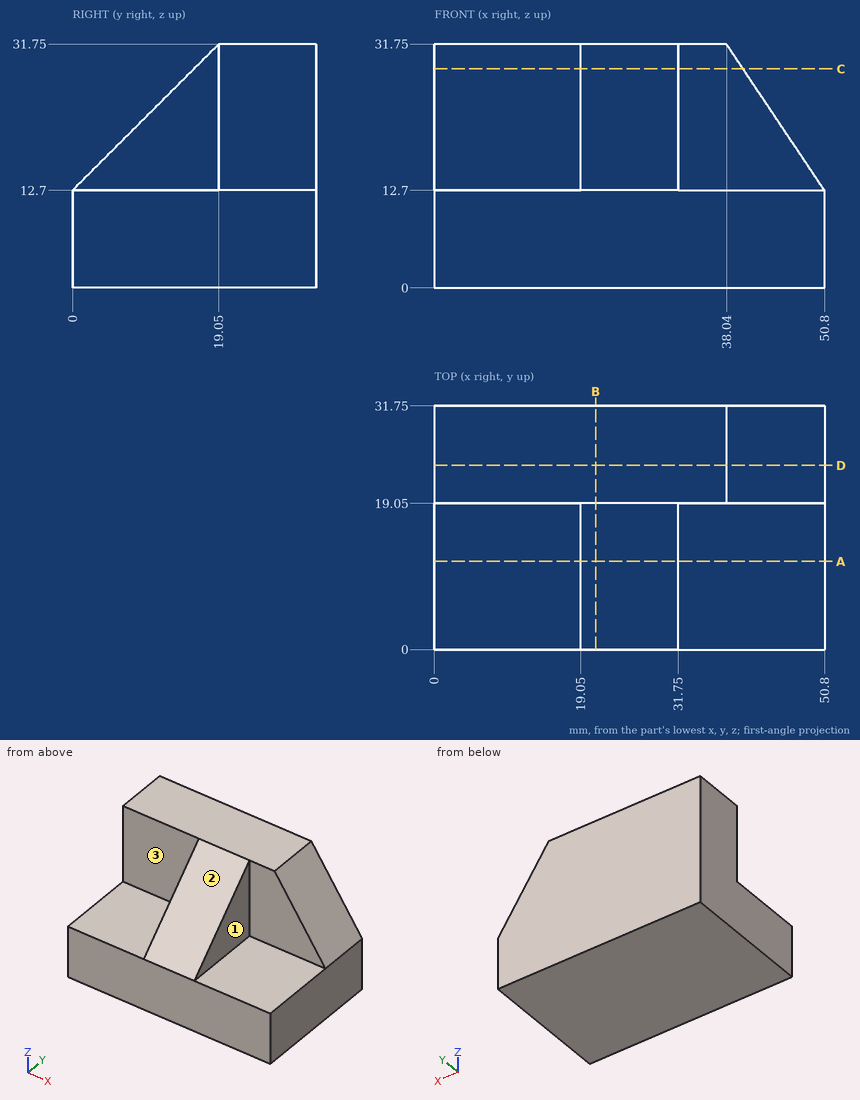
Job drawing, mm, ordinate dimensions from the low corner. One solid piece. A direction names the side the tool comes from. Coordinates: 2 decimals unless noted, no trailing zeros. Write each loop counter-clockwise with the first axis right and the second up, starting at its lowest first coordinate (ties: lowest second). Pieces come first, ordered by that corner, then holes.
Item 1: Pin check, flat tips, straight feed: pin 1 (3 mm diameter, centred on x = 5.5, y = 7, fed in from +Z); pin 2 (9.5 mm diameter, centred on x = 40, z = 20, fed in from -Y); pin 3 (1.5 mm diameter, centred on y = 6.5, z = 13.5, fed in from +X). Stop position of each tip, or through.
Item 2: Which spindle directions (+Z, -Z, +X, -X, +Y, -Y) get a long thin tool onto all of the face, cutting with end or side? Do the marked faces 1, 2 and 3. Say none if no direction does.
Item 3: Slice it at A-A (y = 11.5). Write the cut outline in (x, z), and give its area (3 significant figures).
Item 4: Probe line 1 (Z direction, x = 37.5, y = 8); line 2 (X direction, y = 3.5, z = 15). List the from-to ranges inside material, lowest first.
Item 5: Slice it at C-C (z = 28.5). Write the cut outline in (x, y).
Item 6: Slice it at B-B (x = 21). Write the cut outline in (y, z), and give its area (3 significant figures).
Item 7: Slice it at D-D (y = 24). Write the cut outline in (x, z).
Results found:
1. pin 1: stops at z = 12.7
1. pin 2: stops at y = 19.05
1. pin 3: stops at x = 31.75
2. face 1: +Z, +X, -Y
2. face 2: +Z, +X, -X, -Y
2. face 3: +Z, -X, -Y
3. outline: (0, 0) - (50.8, 0) - (50.8, 12.7) - (31.75, 12.7) - (31.75, 24.2) - (19.05, 24.2) - (19.05, 12.7) - (0, 12.7) - close
3. area: 791 mm2
4. line 1: z = 0 to 12.7
4. line 2: x = 19.05 to 31.75
5. outline: (0, 19.05) - (19.05, 19.05) - (19.05, 15.8) - (31.75, 15.8) - (31.75, 19.05) - (40.22, 19.05) - (40.22, 31.75) - (0, 31.75) - close
6. outline: (0, 0) - (31.75, 0) - (31.75, 31.75) - (19.05, 31.75) - (0, 12.7) - close
6. area: 827 mm2
7. outline: (0, 0) - (50.8, 0) - (50.8, 12.7) - (38.04, 31.75) - (0, 31.75) - close
